from build123d import *

# Parameters (mm, degrees)
F0_W     = 100
F0_H     = 100
F0_R     = 7
F1_DEPTH = 10


with BuildPart() as f1:
    # F0 (on Right) → F1 (new body)
    with BuildSketch(Plane.YZ):
        Rectangle(F0_W, F0_H)
        with Locations((-30, -25.5)):
            Circle(F0_R, mode=Mode.SUBTRACT)
        with Locations((30, -25.5)):
            Circle(F0_R, mode=Mode.SUBTRACT)
        with Locations((-30, 34.5)):
            Circle(F0_R, mode=Mode.SUBTRACT)
        with Locations((30, 34.5)):
            Circle(F0_R, mode=Mode.SUBTRACT)
    extrude(amount=F1_DEPTH)


solid = f1.part
CAD build for the part. Positions are in the model's coordinates, mm. Round coordinates to 2 decimals unless told otherwise and drop trailing zeros. Order: outer loops, then holes, each group sorted by start corner. A loop starts at its lowest first (then second) coordinate and runs counter-clockwise, first axis right, second up. Notation, with made-up numbers: (-7, 78) -> (39, 78) arc R10 ccw to (39, 89) -> close; hole circle Ø11 at (77, 45.25). An arc over 180 degrees is marked (long way). Write each question's results on one line, items separated by ' | '.
1. Cut at A-A (z = -25.5). Give the cut face in (x, y), plus the area to 3 significant figures.
Findings below:
outline: (0, -50) -> (10, -50) -> (10, -37) -> (0, -37) -> close; (0, -23) -> (10, -23) -> (10, 23) -> (0, 23) -> close; (0, 37) -> (10, 37) -> (10, 50) -> (0, 50) -> close | area: 720 mm²
2. Wall check: line 1 along Z through (x, y) = (3.5, 30); line 2 along Z through (x, y) = (2, -33.5). Give the ranges that are in metal, low to high. Write a range as [from, to].
Findings below:
line 1: z = [-50, -32.5], [-18.5, 27.5], [41.5, 50] | line 2: z = [-50, -31.56], [-19.44, 28.44], [40.56, 50]
3. Flat gauge pin, fed straight in: P1, Ø6, axis at y = 1.5, z = -6, coming from the -X side. Where does the tip first touch, or does it go through?
Findings below:
P1: stops at x = 0
4. Pull direction Y, two halves, no side cores. Call faces 1 (the face through (4.93, -26.77, -31.71)), 2 (the face through (5, -50, -1)), 3 (the face through (5, -1, -50)): pulls with the +Y half, pulls with the -Y half, needs draft (parallel to the pull), parting line crosses it, or undercut.
Findings below:
face 1: undercut | face 2: pulls with the -Y half | face 3: needs draft
5. Cut at C-C (y = -30.5). Give the cut face in (x, z), plus the area to 3 significant figures.
Findings below:
outline: (0, -50) -> (10, -50) -> (10, -32.48) -> (0, -32.48) -> close; (0, -18.52) -> (10, -18.52) -> (10, 27.52) -> (0, 27.52) -> close; (0, 41.48) -> (10, 41.48) -> (10, 50) -> (0, 50) -> close | area: 721 mm²
6. Cut at B-B (x = 6). Give the cut face in (y, z).
Findings below:
outline: (-50, -50) -> (50, -50) -> (50, 50) -> (-50, 50) -> close; hole circle Ø14 at (-30, -25.5); hole circle Ø14 at (-30, 34.5); hole circle Ø14 at (30, -25.5); hole circle Ø14 at (30, 34.5)
